Source: CAD feature listing. Evaluate the final solid. Frame: model axes, mm. A direction names the side the tool comes from. Round coordinates to 2 decimals unless told otherwise and drop trailing zeros. Write each loop counter-clockwise with the first axis right and the second up, starting at its lowest first coordinate (ties: lowest second). Pieces come first, ordered by that corner, then holes. Notation, with made-up numbers: M 35.5,-20.5 L 84.5,-20.5 A36 ccw 84.5,15.5 Z; hole C 55.25,42.5 d5. An arc over 180 degrees is marked long. Use a Markdown table: item, result.
```python
from build123d import *

# Parameters (mm, degrees)
F0_R     = 3.175
F1_DEPTH = 1.70942
F2_R     = 3.96875
F3_DEPTH = 3.175
F4_R     = 3.175
F5_DEPTH = 3.175
F6_R     = 2.15265
F7_DEPTH = 119.0625
F8_W     = 3.339038
F8_H     = 0.79375
F9_DEPTH = 14.2875


with BuildPart() as f1:
    # F0 (on Top) → F1 (new body)
    with BuildSketch(Plane.XY):
        Circle(F0_R)
    extrude(amount=F1_DEPTH)

    # F2 (on face) → F3 (join)
    with BuildSketch(Plane.XY.offset(1.70942)):
        Circle(F2_R)
    extrude(amount=F3_DEPTH)

    # F4 (on face) → F5 (join)
    with BuildSketch(Plane.XY.offset(4.88442)):
        Circle(F4_R)
    extrude(amount=F5_DEPTH)

    # F6 (on face) → F7 (join)
    with BuildSketch(Plane.XY.offset(8.05942)):
        Circle(F6_R)
    extrude(amount=F7_DEPTH)

    # F8 (on face) → F9 (cut)
    with BuildSketch(Plane.XY.offset(127.12192)):
        with Locations((0, -1.755775)):
            Rectangle(F8_W, F8_H)
    extrude(amount=-F9_DEPTH, mode=Mode.SUBTRACT)


solid = f1.part
```
Q1. Section B-B on x = 0. Return loops of the section in (y, z) (3 decimals), plus the area to 3 significant figures.
Results are:
| item | result |
|---|---|
| outline | M -3.969,1.709 L -3.175,1.709 L -3.175,0 L 3.175,0 L 3.175,1.709 L 3.969,1.709 L 3.969,4.884 L 3.175,4.884 L 3.175,8.059 L 2.153,8.059 L 2.153,127.122 L -1.359,127.122 L -1.359,112.834 L -2.153,112.834 L -2.153,8.059 L -3.175,8.059 L -3.175,4.884 L -3.969,4.884 Z |
| area | 557 mm^2 |
Q2. First-contact query: pin 1 Ø3 at (x, z) = (0, 54.5) entering from +Y; pin 2 Ø1 at (x, z) = (-0.5, 116.5) entering from -Y; pin 3 Ø4 at (y, z) = (2, 113) entering from -X; pin 4 Ø4 at (x, y) = (-1, -1.5) entering from +Z. Flat tips, straight axial feed; report the tip coordinate or a pass-through.
Results are:
| item | result |
|---|---|
| pin 1 | y = 2.15 |
| pin 2 | y = -1.36 |
| pin 3 | x = -2.15 |
| pin 4 | z = 127.12 |
Q3. Reachability of faces 1 (the cylindrical face through (-0.69, -3.1, 0.84)), 2 (the cylindrical face through (-0.28, 2.134, 66.757)), 3 (the flat face through (0, -1.359, 120)) from +Z, -Z, +X, -X, +Y, -Y: full face, straight path, thin tool, end or side. Return the list, or none.
Results are:
| item | result |
|---|---|
| face 1 | -Z |
| face 2 | +Z |
| face 3 | +Z, +X, -X, -Y |
Q4. Section A-A on y = 0. Return loops of the section in (x, z) (3 decimals), plus the area to 3 significant figures.
Results are:
| item | result |
|---|---|
| outline | M -3.969,1.709 L -3.175,1.709 L -3.175,0 L 3.175,0 L 3.175,1.709 L 3.969,1.709 L 3.969,4.884 L 3.175,4.884 L 3.175,8.059 L 2.153,8.059 L 2.153,127.122 L -2.153,127.122 L -2.153,8.059 L -3.175,8.059 L -3.175,4.884 L -3.969,4.884 Z |
| area | 569 mm^2 |
Q5. Section C-C on z = 31.5. Return loops of the section in (x, y), plus the area to 3 significant figures.
Results are:
| item | result |
|---|---|
| outline | C 0,0 d4.31 |
| area | 14.6 mm^2 |
Q6. Line query: L1, parallel to Y at x = 0.25, z = 38; L2, parallel to Z at x = -0.25, y = 3.25; L3, parallel to Y at x = -0.25, z = 114.5. Output: solid intervals per line, ascending.
Results are:
| item | result |
|---|---|
| L1 | -2.14 to 2.14 |
| L2 | 1.71 to 4.88 |
| L3 | -1.36 to 2.14 |
